Read the model definition and answer for the solid it produces. Units are mm, in the model's axes. A direction names the side the tool comes from. Coordinates: 2 decimals unless noted, no trailing zeros. Loops run counter-clockwise (first coordinate to the right, second up) from the corner with the lowest first, then second, coordinate; pieces in that order, holes last. Notation, with made-up numbers: (22, 82) - (73, 82) arc R18 cw to (73, 112) - close; hole circle Ø8 at (58.25, 11.25). An arc over 180 degrees is marked (long way). Use CSV: the item, a comma, the result in double quotes.
Solid Edge part; units mm, degrees
sketch "Sketch1" plane through (0, 0, 0) normal (0, 0, 1) x (1, 0, 0)
  line L0 (5, -4.2) -> (-5, -4.2)
  line L1 (5, 4.2) -> (-5, 4.2)
  arc A0 (-5, -4.2) -> (-5, 4.2) centre (-5, 0) cw
  arc A1 (5, 4.2) -> (5, -4.2) centre (5, 0) cw
extrude "Protrusion1" add sketch "Sketch1" along normal blind 10
sketch "Sketch2" plane through (0, 0, 0) normal (0, 0, 1) x (1, 0, 0)
  circle A0 centre (5, 0) radius 3
  circle A1 centre (-5, 0) radius 3
extrude "VaciadoExtruido_1" cut sketch "Sketch2" along normal blind 9
sketch "Sketch3" plane through (0, 0, 0) normal (0, 0, 1) x (1, 0, 0)
  circle A0 centre (5, 0) radius 4
  circle A1 centre (-5, 0) radius 4
extrude "VaciadoExtruido_2" cut sketch "Sketch3" along normal blind 1
fillet "Redondeo_1" radius 1.5 2 edges at (2, 0, 9) (-8, 0, 9)
fillet "Redondeo_2" radius 2 4 edges at (-9.2, 0, 10) (9.2, 0, 10) (0, -4.2, 10) (0, 4.2, 10)
sketch "Sketch4" plane through (0, 0, 10) normal (0, 0, 1) x (-1, 0, 0)
  circle A0 centre (-5, 0) radius 0.5
  circle A1 centre (5, 0) radius 0.5
extrude "Cutout1" cut sketch "Sketch4" against normal through all
Q1. The part is cut by section A-A on z = 4.25. Determine the outline of the cut face in (x, y).
Reported:
outline,"(-5, -4.2) - (5, -4.2) arc R4.2 ccw to (5, 4.2) - (-5, 4.2) arc R4.2 ccw to start; hole circle Ø6 at (-5, 0); hole circle Ø6 at (5, 0)"
Q2. The part is cut by section C-C on y = 0. Give the number of separate pieces and of enclosed holes in the cut face, and give its area (3 significant figures).
Reported:
separate pieces,"3"
enclosed holes,"0"
area,"70.2 mm²"
Q3. Find the intervals of material crossed by probe 1 along X at (y, z) = (0, 5.75); probe 2 along X at (y, z) = (1.25, 3); probe 3 along Z at (x, y) = (2.25, 1.5), in increasing order. Write a range as [from, to].
Reported:
probe 1,"x = [-9.2, -8], [-2, 2], [8, 9.2]"
probe 2,"x = [-9.01, -7.73], [-2.27, 2.27], [7.73, 9.01]"
probe 3,"z = [1, 10]"
Q4. For a pull along X with two mould halves and no side action, classify faces 1 (the face through (9.2, 0.1, 3.9)), 2 (the face through (-0.07, -3.63, 9.4)), 3 (the face through (6, 0, 9)) as +X half, -X half, draft (parallel to the pull), parting line (faces both ways), or undercut.
Reported:
face 1,"+X half"
face 2,"draft"
face 3,"undercut"
Q5. The part is cut by section B-B on x = -0.25. Determine the outline of the cut face in (y, z), and give its area (3 significant figures).
Reported:
outline,"(-4.2, 0) - (4.2, 0) - (4.2, 8) arc R2 ccw to (2.2, 10) - (-2.2, 10) arc R2 ccw to (-4.2, 8) - close"
area,"82.3 mm²"
Q6. The part is cut by section D-D on z = 9.25. Determine the outline of the cut face in (x, y), and give its area (3 significant figures).
Reported:
outline,"(-5, -3.76) - (5, -3.76) arc R3.76 ccw to (5, 3.76) - (-5, 3.76) arc R3.76 ccw to start; hole circle Ø1 at (-5, 0); hole circle Ø1 at (5, 0)"
area,"118 mm²"
Q7. A tool of negligible diameter and unlimited length cuts with its end or side. For faces 4 (the face through (6, 3, 1)), 5 (the face through (-9.2, -0.1, 3.9)), from which of +Z, -Z, +X, -X, +Y, -Y can it reach the whole face along a straight path? Write none if from no direction.
Reported:
face 4,"-Z"
face 5,"+Z, -Z, -X"
Q8. Given P1, Ø1, axis at y = 2.5, z = 8.5, coming from the -X side; P2, Ø1.5, axis at x = 5, y = 0.5, coming from the -Z side; P3, Ø3, axis at x = 5, y = 2, coming from the -Z side, each flat-ended and moving along its own axis, determine where each tip first touches the part or whether it passes through.
Reported:
P1,"stops at x = -8.65"
P2,"stops at z = 9"
P3,"stops at z = 1"
